```python
from build123d import *

# Parameters (mm, degrees)
PAD_DEPTH               = 10
PADBODY_PLACEMENT_ANGLE = 90


with BuildPart() as part:
    # Sketch → Pad (new body)
    with BuildSketch(Plane.XY):
        Polygon((0, 0), (54.3, 0), (79.777916, 70), (54.3, 80), (0, 80), align=None)
    extrude(amount=PAD_DEPTH)


with BuildPart() as part_1:
    # PadBody placement: moved
    add(part.part.rotate(Axis((0, 0, 0), (1, 0, 0)), PADBODY_PLACEMENT_ANGLE))


solid = part_1.part
```
Check sheet for the modelled part. Datum: model origin and axes. Units: mm. Round coordinates to 2 decimals unless told otherwise and drop trailing zeros. Order: outer loops, then holes, each group sorted by start corner. A loop starts at its lowest first (then second) coordinate and runs counter-clockwise, first axis right, second up. Notation, with made-up numbers: (27.5, 87.25) - (70.5, 87.25) arc R11 cw to (70.5, 91.25) - close; hole circle Ø9 at (22.5, 51.25). An arc over 180 degrees is marked (long way). Write item = value, one per line.
Q1. Section check C-C (z = 58). Record the boundary of the cut face in (x, y).
Computed:
outline = (0, -10) - (75.41, -10) - (75.41, 0) - (0, 0) - close
Q2. Section check A-A (y = -7). Record the boundary of the cut face in (x, z), and give its area (3 significant figures).
Computed:
outline = (0, 0) - (54.3, 0) - (79.78, 70) - (54.3, 80) - (0, 80) - close
area = 5,360 mm^2
Q3. Section check B-B (x = 72.5). Record the boundary of the cut face in (y, z), and give its area (3 significant figures).
Computed:
outline = (-10, 50) - (0, 50) - (0, 72.86) - (-10, 72.86) - close
area = 229 mm^2
Q4. Go/stop test with flat-tipped pins: pin 1 (1 mm diameter, centred on y = -5, z = 42.5, fed in from +X); pin 2 (1 mm diameter, centred on y = -1, z = 10.5, fed in from +X). Record where each tip stops, or that it passes through.
Computed:
pin_1 = 69.95
pin_2 = 58.3
Q5. Thickness scan on line 1 along X through (y, z) = (-2.25, 64); line 2 along X through (y, z) = (-6, 46). Record the ranges inside material, lowest first.
Computed:
line_1 = 0 to 77.59
line_2 = 0 to 71.04
